Model file for the job. Use its own axes, mm. Face numbers are marked on the shaded views. Give positions to 0.01 mm unless a question says otherwise; leave off trailing zeros. Write each loop counter-clockwise with the first axis right and the second up, starting at its lowest first coordinate (ties: lowest second). Pieces come first, ordered by that corner, then holes.
```python
from build123d import *

# Parameters (mm, degrees)
F0_R     = 9.5
F1_DEPTH = 3
F2_R     = 0.5
F7_D     = 15


with BuildPart() as f1:
    # F0 (on Top) → F1 (new body)
    with BuildSketch(Plane.XY):
        Circle(F0_R)
    extrude(amount=F1_DEPTH)

    # F5: sweep along a path in F4
    with BuildLine(Plane.XY.offset(1)) as f5_path:
        CenterArc((0, 0), 9.5, 0, 360)
    # F2 (on Front) → F5 (sweep, cut)
    with BuildSketch(Plane.XZ):
        with Locations((9.5, 1)):
            Circle(F2_R)
    sweep(path=f5_path.line, mode=Mode.SUBTRACT)

    # F7 (through all)
    with Locations(Plane(origin=(0, 0, 0), x_dir=(1, 0, 0), z_dir=(0, 0, -1))):
        with Locations((0, 0)):
            Hole(F7_D / 2)


solid = f1.part
```
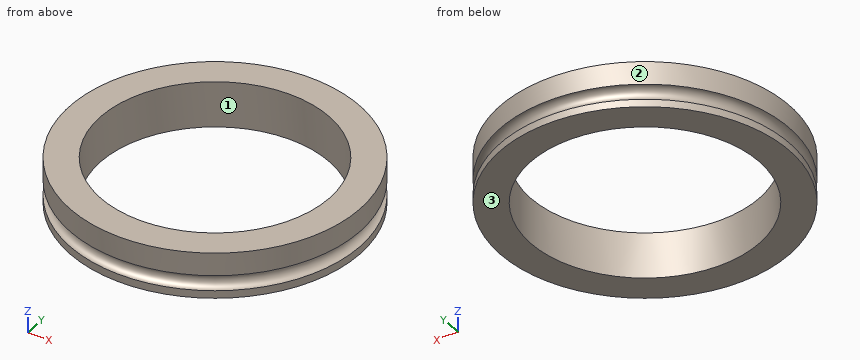
1. Slice it at C-C, the plane z = 1.75. Write the cut outline in (x, y).
Calculated:
outline: circle Ø19 at (0, 0); hole circle Ø15 at (0, 0)
2. Slice it at A-A, the plane x = 0. Write the cut outline in (y, z), and give its area (3 significant figures).
Calculated:
outline: (-9.5, 0) - (-7.5, 0) - (-7.5, 3) - (-9.5, 3) - (-9.5, 1.5) arc R0.5 cw to (-9.5, 0.5) - close; (7.5, 0) - (9.5, 0) - (9.5, 0.5) arc R0.5 cw to (9.5, 1.5) - (9.5, 3) - (7.5, 3) - close
area: 11.2 mm2
3. Pin check, flat tips, straight feed: P1, Ø1.5, axis at x = 6.5, z = 1, coming from the -Y side; P2, Ø1, axis at x = 4, z = 0.5, coming from the +Y side. Stop position of each tip, or through.
Calculated:
P1: stops at y = -7.41
P2: stops at y = 8.83
4. Probe probe 1 along Y at (x, z) = (0, 2.45); probe 2 along X at (y, z) = (-3, 1.95); probe 3 along Y at (x, z) = (0, 0.85). List the from-to ranges inside material, lowest first.
Calculated:
probe 1: y = -9.5 to -7.5, 7.5 to 9.5
probe 2: x = -9.01 to -6.87, 6.87 to 9.01
probe 3: y = -9.02 to -7.5, 7.5 to 9.02
5. Pull direction X, two halves, no side cores. Call the marked faces 1, 2 and 3: +X half, -X half, draft (parallel to the pull), parting line (faces both ways), or undercut.
Calculated:
face 1: undercut
face 2: parting line
face 3: draft
